Geometry check sheet. Reference: the model listing, model coordinates, mm. A direction names the side the tool comes from. Round coordinates to 2 decimals unless told otherwise and drop trailing zeros. Write each loop counter-clockwise with the first axis right and the second up, starting at its lowest first coordinate (ties: lowest second). Pieces come first, ordered by that corner, then holes.
Item 1: Cross-section at A-A (z = 5). Enter the section's corners in (x, y).
Item 2: Draft check along X on faces 4 (the face through (29.454, 11.837, 5.066)), 5 (the face through (-4.524, 1, 5)), 6 (the face through (1.475, -1, 5)), 7 (the face through (19, 10.358, 5)). Enter one of: pulls with the +X half, pulls with the -X half, needs draft (parallel to the pull), parting line crosses it, or undercut.
Item 3: Cross-section at B-B (y = 12). Enter the section's corners in (x, z), then the cut area to 3 significant figures.
Item 4: Cross-section at D-D (y = -0.75). Enter the section's corners in (x, z).
Item 5: Scan lines: probe 1 along Y at (x, z) = (12, 9); probe 2 along Y at (x, z) = (38, 9.25); probe 3 along X at (y, z) = (-1.75, 2.5). Record each from-to range of solid material in increasing order.
Item 6: Cross-section at C-C (x = 38). Enter the section's corners in (y, z).
Item 7: Depth check by flat-ended pin: P1, Ø3, axis at x = 1.5, z = 7.5, coming from the +Y side; P2, Ø6, axis at x = 16.5, z = 7, coming from the +Y side; P3, Ø1.6, axis at x = 30.5, z = 4, coming from the +Y side. Enter the tip coordinate at first touch or a pass-through.
Item 8: Access from +Z, -Z, +X, -X, +Y, -Y to the whole of each face (thin tool, end or side, straight path). Record for faces 1 (the face through (40.038, 9.907, 5.231)), 2 (the face through (13, 7, 10)), 3 (the face through (28.685, 11.837, 4.916)).
from build123d import *

# Parameters (mm, degrees)
BOSS_EXTRUDE1_DEPTH = 10
BOSS_EXTRUDE4_DEPTH = 8
SKETCH7_R           = 5.25
CUT_EXTRUDE1_DEPTH  = 7
SKETCH8_W           = 10
SKETCH8_H           = 4
BOSS_EXTRUDE5_DEPTH = 11
CUT_EXTRUDE2_DEPTH  = 10
BOSS_EXTRUDE6_DEPTH = 3
BOSS_EXTRUDE7_DEPTH = 10
CUT_EXTRUDE3_DEPTH  = 10
SKETCH13_W          = 5.998509049
SKETCH13_H          = 10
BOSS_EXTRUDE8_DEPTH = 3


with BuildPart() as part:
    # Sketch2 → Boss-Extrude1 (new body)
    with BuildSketch(Plane.XY):
        Polygon((6.476, 10.358), (31.476, 10.358), (31.476, 5.358), (11.456, 5.358), (11.456, 0), (6.476, 0), align=None)
    extrude(amount=BOSS_EXTRUDE1_DEPTH)

    # Sketch6 → Boss-Extrude4 (add)
    with BuildSketch(Plane.XZ.offset(-5.358)):
        with BuildLine():
            Line((31.476, 0), (31.476, 10))
            ThreePointArc((31.476, 10), (40.79262479, 5), (31.476, 0))
        make_face()
    extrude(amount=-BOSS_EXTRUDE4_DEPTH)

    # Sketch7 → Cut-Extrude1 (cut)
    with BuildSketch(Plane(origin=(0, 13.358, 0), x_dir=(1, 0, 0), z_dir=(0, 1, 0))):
        with Locations(Location((34.79262479, -5, 0), (0, 0, 180))):
            Circle(SKETCH7_R)
    extrude(amount=-CUT_EXTRUDE1_DEPTH, mode=Mode.SUBTRACT)

    # Sketch8 → Boss-Extrude5 (add)
    with BuildSketch(Plane.ZY.offset(-6.476)):
        with Locations((5, 2)):
            Rectangle(SKETCH8_W, SKETCH8_H)
    extrude(amount=BOSS_EXTRUDE5_DEPTH)

    # Sketch9 → Cut-Extrude2 (cut)
    with BuildSketch(Plane.XY.offset(10)):
        Polygon((11.456, 5.358), (6.259030685, 0), (11.456, 0), align=None)
    extrude(amount=-CUT_EXTRUDE2_DEPTH, mode=Mode.SUBTRACT)

    # Sketch10 → Boss-Extrude6 (add)
    with BuildSketch(Plane(origin=(0, 10.358, 0), x_dir=(1, 0, 0), z_dir=(0, 1, 0))):
        with BuildLine():
            Line((31.476, -10), (31.476, -9.069705149))
            ThreePointArc((31.476, -9.069705149), (29.453104981, -5), (31.476, -0.930294851))
            Line((31.476, -0.930294851), (31.476, 0))
            ThreePointArc((31.476, 0), (28.684587845, -5), (31.476, -10))
        make_face()
    extrude(amount=BOSS_EXTRUDE6_DEPTH)

    # Sketch11 → Boss-Extrude7 (add)
    with BuildSketch(Plane.XY.offset(10)):
        Polygon((6.476, 4), (6.476, 10.358), (0.118, 4), align=None)
    extrude(amount=-BOSS_EXTRUDE7_DEPTH)

    # Sketch12 → Cut-Extrude3 (cut)
    with BuildSketch(Plane.XY.offset(10)):
        Polygon((6.259030685, 0), (1.474509049, 0), (6.671478364, 5.358), (11.456, 5.358), align=None)
    extrude(amount=-CUT_EXTRUDE3_DEPTH, mode=Mode.SUBTRACT)

    # Sketch13 → Boss-Extrude8 (add)
    with BuildSketch(Plane.XZ):
        with Locations((-1.524745476, 5)):
            Rectangle(SKETCH13_W, SKETCH13_H)
    extrude(amount=BOSS_EXTRUDE8_DEPTH)


solid = part.part
Resolved:
1. outline: (-4.52, -3) - (1.47, -3) - (1.47, 0) - (6.67, 5.36) - (40.79, 5.36) - (40.79, 13.36) - (40.04, 13.36) - (40.04, 6.36) - (29.54, 6.36) - (29.54, 10.36) - (29.45, 10.36) - (29.45, 13.36) - (28.68, 13.36) - (28.68, 10.36) - (6.48, 10.36) - (0.12, 4) - (-4.52, 4) - close
2. face 4: undercut
2. face 5: pulls with the -X half
2. face 6: pulls with the +X half
2. face 7: needs draft
3. outline: (31.48, 0) arc R6 ccw (long way) to (31.48, 10) arc R5.87 ccw to start; hole (31.48, 0.93) arc R5.25 ccw (long way) to (31.48, 9.07) arc R5.11 ccw to start
3. area: 26.8 mm2
4. outline: (-4.52, 0) - (1.47, 0) - (1.47, 10) - (-4.52, 10) - close
5. probe 1: y = 5.36 to 10.36
5. probe 2: y = 5.36 to 13.36
5. probe 3: x = -4.52 to 1.47
6. outline: (5.36, -0.07) - (13.36, -0.07) - (13.36, 0.84) - (6.36, 0.84) - (6.36, 9.16) - (13.36, 9.16) - (13.36, 10.07) - (5.36, 10.07) - close
7. P1: stops at y = 6.88
7. P2: stops at y = 10.36
7. P3: stops at y = 6.36
8. face 1: +Y
8. face 2: +Z, -X, +Y, -Y
8. face 3: -X, +Y
